Here's the drawing with two shaded views (mm, measured from the low corner). I have some questions. A direction names the side the tool comes from. Round coordinates to 2 decimals unless told otherwise and drop trailing zeros. Order: outer loops, then holes, each group sorted by start corner. A loop starts at its lowest first (then second) coordinate and runs counter-clockwise, first axis right, second up. Notation, with made-up numbers: (55.25, -29.75) -> (103.25, -29.75) arc R25 cw to (103.25, -15.75) -> close; hole circle Ø11 at (34.5, 11.25). An arc over 180 degrees is marked (long way). Use a Markdown table: item, result. Add a question column.
Q1. If we section it at C-C on z = 22.5: List the corners of the cut face in (x, y) for me, plus the area to 3 significant figures.
Q2. I'm going to push flat-ended pins straight in: pin 1 Ø7.5 at (x, z) = (7, 50) entering from +Y; pin 2 Ø16.5 at (x, y) = (11, 22.5) entering from -Z; pin 3 Ø8 at (x, y) = (80, 22.5) entering from -Z (3 decimals); pin 4 Ø2.5 at (y, z) = (64, 91.5) entering from -X. Where does each tip first touch, or does it pass through?
Q3. For the marked faces 4, 5 and 6, which set-ups out of +Z, -Z, +X, -X, +Y, -Y let a thin tool reach every point of the face, with its end or its side?
Q4. If we section it at B-B on x = 80: List the corners of the cut face in (y, z) for me, plus the area to 3 significant figures.
Q5. We'd pull the mould along Z, two halves only. Please class the marked faces 1, 2 and 3: +Z half, -Z half, draft (parallel to the pull), parting line (faces both ways), or undercut.
Q6. If we section it at D-D on y = 32: List the corners of the cut face in (x, z) for me, plus the area to 3 significant figures.
Q7. If we section it at A-A on y = 22.5: Give the number of separate pieces and of enclosed holes in the cut face, plus the area to 3 significant figures.
Q8. I need wall thicknesses on line 1 along Z through (x, y) = (92.5, 22); line 2 along Z through (x, y) = (65.5, 11). Which ranges of each line are inside material? Lowest first, please. Write a range as [from, to].
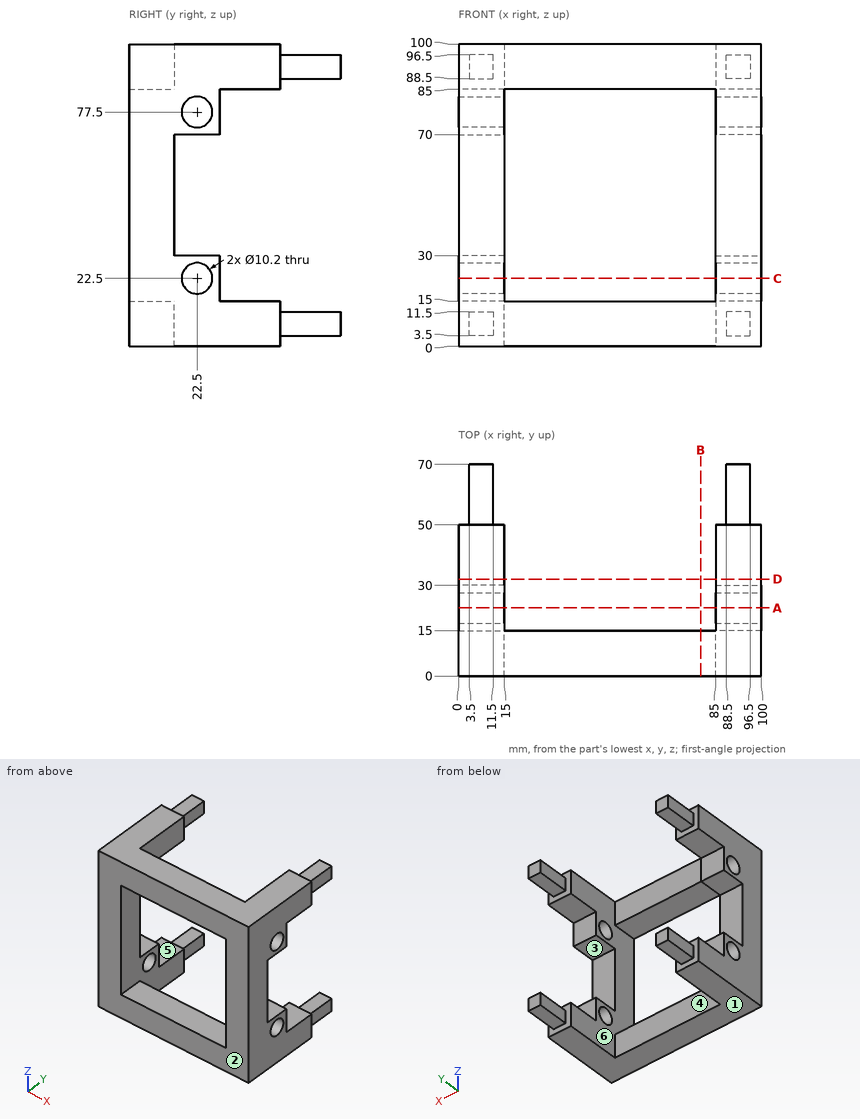
Answer below:
| question | item | result |
|---|---|---|
| 1 | outline | (0, 0) -> (15, 0) -> (15, 17.4) -> (0, 17.4) -> close; (0, 27.6) -> (15, 27.6) -> (15, 30) -> (0, 30) -> close; (85, 0) -> (100, 0) -> (100, 17.4) -> (85, 17.4) -> close; (85, 27.6) -> (100, 27.6) -> (100, 30) -> (85, 30) -> close |
| 1 | area | 594 mm² |
| 2 | pin 1 | y = 15 |
| 2 | pin 2 | z = 0 |
| 2 | pin 3 | through |
| 2 | pin 4 | x = 3.5 |
| 3 | face 4 | +Z, -Z, +Y |
| 3 | face 5 | +X, -X, +Y |
| 3 | face 6 | +Y |
| 4 | outline | (0, 0) -> (15, 0) -> (15, 15) -> (0, 15) -> close; (0, 85) -> (15, 85) -> (15, 100) -> (0, 100) -> close |
| 4 | area | 450 mm² |
| 5 | face 1 | -Z half |
| 5 | face 2 | draft |
| 5 | face 3 | undercut |
| 6 | outline | (0, 0) -> (15, 0) -> (15, 15) -> (0, 15) -> close; (0, 85) -> (15, 85) -> (15, 100) -> (0, 100) -> close; (85, 0) -> (100, 0) -> (100, 15) -> (85, 15) -> close; (85, 85) -> (100, 85) -> (100, 100) -> (85, 100) -> close |
| 6 | area | 900 mm² |
| 7 | separate pieces | 8 |
| 7 | enclosed holes | 0 |
| 7 | area | 1,190 mm² |
| 8 | line 1 | [0, 17.42], [27.58, 30], [70, 72.42], [82.58, 100] |
| 8 | line 2 | [0, 15], [85, 100] |
